Here's how the part is built. I have some questions about the finished solid (model axes, mm). Round coordinates to 2 decimals unless told otherwise and drop trailing zeros. Write each loop counter-clockwise with the first axis right and the second up, starting at its lowest first coordinate (ties: lowest second). Pieces come first, ordered by that corner, then holes. Notation, with made-up numbers: M 54.25,86.5 L 112.25,86.5 A30 ccw 112.25,118.5 Z; hole C -36.5,-12 d11. An arc over 180 degrees is marked long. Use one line per item in the form item = value. Start each with the question number.
Q1. I'm going to push flat-ended pins straight in: pin 1 Ø1.6 at (x, z) = (2, -21.5) entering from -Y; pin 2 Ø1.5 at (y, z) = (-111.5, 19) entering from -X; pin 3 Ø0.9 at (x, y) = (2, -129) entering from -Z. Where does each tip first touch, or does it pass through?
Q2. I need wall thicknesses on line 1 along Y through (x, z) = (2.25, -22.5); line 2 along Z through (x, y) = (1.25, -111); line 3 along Y through (x, z) = (1.7, 22). Which ranges of each line are inside material? Lowest first, please. Write a range as from..to.
Q3. I want a section at A-A on x = 2.5. List the corners of the cut face in (y, z) for me.
Q4. I want a section at B-B on y = -116. List the corners of the cut face in (x, z) for me, and give its area (3 significant figures).
```python
from build123d import *

# Parameters (mm, degrees)
BOSS_EXTRUDE1_DEPTH = 3
SKETCH2_R           = 0.75
CUT_EXTRUDE1_DEPTH  = 146.674630793
CUT_EXTRUDE2_DEPTH  = 10
FILLET1_R           = 5
FILLET2_R           = 5


with BuildPart() as part:
    # Sketch1 → Boss-Extrude1 (new body)
    with BuildSketch(Plane(origin=(0, 0, 0), x_dir=(0, 0, -1), z_dir=(1, 0, 0))):
        with BuildLine():
            Line((-30, -97.52051802), (-30, -109.52051802))
            ThreePointArc((-30, -109.52051802), (-27.656854249, -115.177372269), (-22, -117.52051802))
            Line((-22, -117.52051802), (-21.5, -117.52051802))
            ThreePointArc((-21.5, -117.52051802), (-18.671572875, -118.692090895), (-17.5, -121.52051802))
            Line((-17.5, -121.52051802), (-17.5, -139.52051802))
            ThreePointArc((-17.5, -139.52051802), (-16.621320344, -141.641838363), (-14.5, -142.52051802))
            Line((-14.5, -142.52051802), (14.5, -142.52051802))
            ThreePointArc((14.5, -142.52051802), (16.621320344, -141.641838363), (17.5, -139.52051802))
            Line((17.5, -139.52051802), (17.5, -121.52051802))
            ThreePointArc((17.5, -121.52051802), (18.671572875, -118.692090895), (21.5, -117.52051802))
            Line((21.5, -117.52051802), (22, -117.52051802))
            ThreePointArc((22, -117.52051802), (27.656854249, -115.177372269), (30, -109.52051802))
            Line((30, -109.52051802), (30, -97.52051802))
            Line((30, -97.52051802), (-30, -97.52051802))
        make_face()
    extrude(amount=BOSS_EXTRUDE1_DEPTH)

    # Sketch2 → Cut-Extrude1 (cut, through all)
    with BuildSketch(Plane(origin=(3, 0, 0), x_dir=(0, 0, -1), z_dir=(1, 0, 0))):
        with Locations((-22.5, -103.52051802)):
            Circle(SKETCH2_R)
        with Locations(Location((-22.5, -111.52051802, 0), (0, 0, 180))):
            Circle(SKETCH2_R)
        with Locations((22.5, -111.52051802)):
            Circle(SKETCH2_R)
        with Locations(Location((22.5, -103.52051802, 0), (0, 0, 180))):
            Circle(SKETCH2_R)
    extrude(amount=-CUT_EXTRUDE1_DEPTH, mode=Mode.SUBTRACT)

    # Sketch3 → Cut-Extrude2 (cut)
    with BuildSketch(Plane(origin=(3, 0, 0), x_dir=(0, 0, -1), z_dir=(1, 0, 0))):
        with BuildLine():
            Line((-30, -97.52051802), (-25, -97.52051802))
            Line((-25, -97.52051802), (-25, -113.936716507))
            ThreePointArc((-25, -113.936716507), (-24.121320344, -116.05803685), (-22, -116.936716507))
            Line((-22, -116.936716507), (-20.5, -116.936716507))
            ThreePointArc((-20.5, -116.936716507), (-18.378679656, -117.815396163), (-17.5, -119.936716507))
            Line((-17.5, -119.936716507), (-17.5, -122.452918804))
            Line((-17.5, -122.452918804), (-42.892449252, -122.452918804))
            Line((-42.892449252, -122.452918804), (-42.892449252, -97.52051802))
            Line((-42.892449252, -97.52051802), (-30, -97.52051802))
        make_face()
        with BuildLine():
            Line((20.5, -116.936716507), (22, -116.936716507))
            ThreePointArc((22, -116.936716507), (24.121320344, -116.05803685), (25, -113.936716507))
            Line((25, -113.936716507), (25, -97.52051802))
            Line((25, -97.52051802), (30, -97.52051802))
            Line((30, -97.52051802), (42.892449252, -97.52051802))
            Line((42.892449252, -97.52051802), (42.892449252, -122.452918804))
            Line((42.892449252, -122.452918804), (17.5, -122.452918804))
            Line((17.5, -122.452918804), (17.5, -119.936716507))
            ThreePointArc((17.5, -119.936716507), (18.378679656, -117.815396163), (20.5, -116.936716507))
        make_face()
    extrude(amount=-CUT_EXTRUDE2_DEPTH, mode=Mode.SUBTRACT)

    # Fillet1
    fillet1_edges = [part.edges().sort_by_distance(p)[0] for p in [
        (1.5, -97.52051802, 25),
    ]]
    fillet(fillet1_edges, radius=FILLET1_R)

    # Fillet2
    fillet2_edges = [part.edges().sort_by_distance(p)[0] for p in [
        (1.5, -97.52051802, -25),
    ]]
    fillet(fillet2_edges, radius=FILLET2_R)


solid = part.part
```
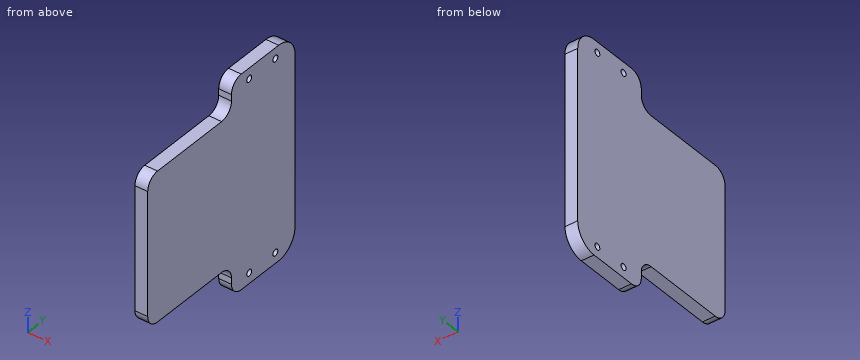
Reported:
q1.pin_1 = -116.94
q1.pin_2 = 0
q1.pin_3 = -17.5
q2.line_1 = -116.89..-112.27, -110.77..-104.27, -102.77..-98.19
q2.line_2 = -25..-23.04, -21.96..21.96, 23.04..25
q2.line_3 = -116.94..-112.08, -110.96..-104.08, -102.96..-97.94
q3.outline = M -142.52,-14.5 A3 ccw -139.52,-17.5 L -119.94,-17.5 A3 cw -116.94,-20.5 L -116.94,-22 A3 ccw -113.94,-25 L -102.52,-25 A5 ccw -97.52,-20 L -97.52,20 A5 ccw -102.52,25 L -113.94,25 A3 ccw -116.94,22 L -116.94,20.5 A3 cw -119.94,17.5 L -139.52,17.5 A3 ccw -142.52,14.5 Z; hole C -111.52,-22.5 d1.5; hole C -111.52,22.5 d1.5; hole C -103.52,-22.5 d1.5; hole C -103.52,22.5 d1.5
q4.outline = M 0,-24.18 L 3,-24.18 L 3,24.18 L 0,24.18 Z
q4.area = 145 mm^2
